Here's how the part is built. I have some questions about the finished solid (model axes, mm). Round coordinates to 2 decimals unless told otherwise and drop trailing zeros. Write each loop counter-clockwise with the first axis right and the second up, starting at its lowest first coordinate (ties: lowest second). Pieces come first, ordered by that corner, then holes. Notation, with made-up numbers: M 37,61 L 71,61 A25 cw 71,84 Z; hole C 40.25,20.25 d5. An arc over 180 degrees is marked long. Write item = value, one per line. Start each with the question number.
(1) I need wall thicknesses on line 1 along X through (y, z) = (-1.95, 35); line 2 along Z through (x, y) = (-58.5, -1.65). Which ranges of each line are inside material? Lowest first, please.
(2) Will these pins go through, and if not, where does the flat tip stop? pin 1 Ø1.5 at (y, z) = (-2, 147.5) entering from -X; pin 2 Ø1.5 at (x, y) = (20, -2) entering from +Z.
(3) I want a section at A-A (z = -17.5). List the corners of the cut face in (x, y) for me, and give its area (3 significant figures).
```python
from build123d import *

# Parameters (mm, degrees)
F0_W     = 70
F0_H     = 3
F1_DEPTH = 3


with BuildPart() as f1:
    # F0 (on Front) → F1 (new body)
    with BuildSketch(Plane.XZ):
        Polygon((-56.857143, 146.714286), (-81.857143, 146.714286), (-81.857143, -53.285714), (-71.857143, -53.285714), (-71.857143, 46.714286), (-68.857143, 46.714286), (-68.857143, -53.285714), (118.142857, -53.285714), (118.142857, -43.285714), (118.142857, -40.285714), (118.142857, 146.714286), (93.142857, 146.714286), (23.142857, 146.714286), (13.142857, 146.714286), align=None)
        with Locations((-21.857143, 148.214286)):
            Rectangle(F0_W, F0_H)
        with Locations((58.142857, 148.214286)):
            Rectangle(F0_W, F0_H)
    extrude(amount=F1_DEPTH)


solid = f1.part
```
Returned:
q1.line_1 = -81.86 to -71.86, -68.86 to 118.14
q1.line_2 = -53.29 to 146.71
q2.pin_1 = -56.86
q2.pin_2 = 146.71
q3.outline = M -81.86,-3 L -71.86,-3 L -71.86,0 L -81.86,0 Z; M -68.86,-3 L 118.14,-3 L 118.14,0 L -68.86,0 Z
q3.area = 591 mm²
